Verification items for the finished model (mm, model axes). A direction names the side the tool comes from. Coordinates: 2 decimals unless noted, no trailing zeros. Loops run counter-clockwise (first coordinate to the right, second up) from the corner with the lowest first, then second, coordinate; pieces in that order, holes last.
Q1. Go/stop test with flat-tipped pins: P1, Ø6, axis at y = -13, z = 25, coming from the -X side; P2, Ø8, axis at x = -11.5, z = 9, coming from the +Y side; P3, Ø6, axis at y = -8, z = 6, coming from the -X side. Record where each tip stops, or that it passes through.
Q2. Material ranges on probe 1 along Z at (x, y) = (13, 11.5); probe 2 along X at (y, z) = (-8, 7.5); probe 3 along Y at (x, z) = (7.5, 16.5), recorded low to high.
Q3. Mould release check, pull along Z, two halves, no side actions. Record for faces 4 (the face through (0, 0, 0)), 5 (the face through (15.653, 6.49, 3.635)), 6 (the face through (6, -16, 21.659)), 7 (the face through (8.767, -16.856, 7.678)): +Z half, -Z half, draft (parallel to the pull), parting line (faces both ways), or undercut.
Q4. Access from +Z, -Z, +X, -X, +Y, -Y to the whole of each face (thin tool, end or side, straight path). Record for faces 1 (the face through (17, 3, 6.1)), 2 (the face through (15.738, -4.956, 25.381)), 3 (the face through (0, 0, 29)).
Q5. Sectioned sample at C-C (z = 25). Enter the section's corners in (x, y).
Q6. Sectioned sample at D-D (z = 10). Enter the section's corners in (x, y) (3 decimals), then the cut area to 3 significant figures.
```python
from build123d import *

# Parameters (mm, degrees)
F0_R     = 19
F1_DEPTH = 29
F2_W     = 13.055
F2_H     = 5
F2_H_2   = 3.12
F2_W_2   = 13.499867
F2_H_3   = 4.67
F2_W_3   = 13.901473
F2_H_4   = 10


with BuildPart() as f1:
    # F0 (on Top) → F1 (new body)
    with BuildSketch(Plane.XY):
        Circle(F0_R)
    extrude(amount=F1_DEPTH)

    # F2 (on Front) → F3 (revolve, cut)
    with BuildSketch(Plane.XZ):
        with Locations((23.4725, 3.6)):
            Rectangle(F2_W, F2_H)
        with Locations((23.4725, 10.86)):
            Rectangle(F2_W, F2_H_2)
        with Locations((23.250066, 16.255)):
            Rectangle(F2_W_2, F2_H_3)
        with Locations((23.450869, 26.65892)):
            Rectangle(F2_W_3, F2_H_4)
    revolve(axis=Axis((0, 0, 8.831585), (0, 0, -1)), mode=Mode.SUBTRACT)


solid = f1.part
```
Geometry check:
1. P1: stops at x = -13.12
1. P2: stops at y = 17.46
1. P3: stops at x = -18.33
2. probe 1: z = 0 to 1.1, 6.1 to 9.3, 12.42 to 13.92, 18.59 to 21.66
2. probe 2: x = -17.23 to 17.23
2. probe 3: y = -14.7 to 14.7
3. face 4: -Z half
3. face 5: undercut
3. face 6: +Z half
3. face 7: draft
4. face 1: none
4. face 2: +Z
4. face 3: +Z, +X, -X, +Y, -Y
5. outline: circle Ø33 at (0, 0)
6. outline: circle Ø33.89 at (0, 0)
6. area: 902 mm2
